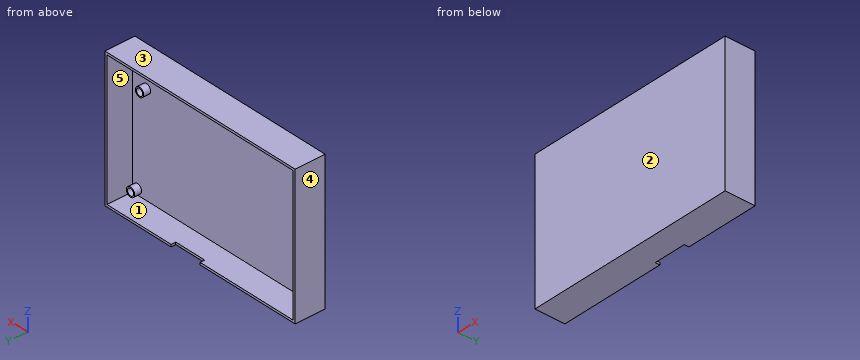
Autodesk Inventor part; units mm, degrees
ref_plane "YZ Plane" through (0, 0, 0) normal (1, 0, 0) x (0, 1, 0)
ref_plane "XZ Plane" through (0, 0, 0) normal (0, 1, 0) x (-1, 0, 0)
ref_plane "XY Plane" through (0, 0, 0) normal (0, 0, 1) x (1, 0, 0)
sketch "Base" plane through (0, 0, 0) normal (0, 1, 0) x (-1, 0, 0)
  line L0 (92, 60.5) -> (-92, 60.5)
  line L1 (-92, 60.5) -> (-92, -60.5)
  line L2 (-92, -60.5) -> (92, -60.5)
  line L3 (92, -60.5) -> (92, 60.5)
  line L4 (92, 60.5) -> (-92, -60.5) construction
  line L5 (-92, 60.5) -> (92, -60.5) construction
  point P0 (0, 0)
  dimension "d0" = 184
  dimension "d1" = 121
extrude "Base - Estrutura" add sketch "Base" against normal blind 26
sketch "Esboço2" plane through (0, 0, 0) normal (0, 1, 0) x (1, 0, 0)
  line L0 (-90, -58.5) -> (90, -58.5)
  line L1 (90, -58.5) -> (90, 58.5)
  line L2 (90, 58.5) -> (-90, 58.5)
  line L3 (-90, 58.5) -> (-90, -58.5)
  line L4 (-90, -58.5) -> (90, 58.5) construction
  line L5 (90, -58.5) -> (-90, 58.5) construction
  point P0 (0, 0)
  dimension "d4" = 180
  dimension "d5" = 117
extrude "Base Interna" cut sketch "Esboço2" against normal blind 22
sketch "Esboço3" plane through (0, -22, 0) normal (0, 1, 0) x (1, 0, 0)
  circle A0 centre (-85, -53.5) radius 4
  line L0 (-92, 60.5) -> (-92, -60.5)
  line L1 (-92, -60.5) -> (92, -60.5)
  circle A1 centre (-85, -53.5) radius 3
  line L2 (-90, -58.5) -> (-90, 58.5)
  line L3 (90, 58.5) -> (90, -58.5)
  circle A2 centre (-85, 53.5) radius 4
  circle A3 centre (-85, 53.5) radius 3
  line L4 (-90, 58.5) -> (90, 58.5)
  line L5 (90, -58.5) -> (-90, -58.5)
  circle A4 centre (85, 53.5) radius 3
  circle A5 centre (85, 53.5) radius 4
  line L6 (92, -60.5) -> (92, 60.5)
  line L7 (92, 60.5) -> (-92, 60.5)
  circle A6 centre (76.27, -28.99) radius 4
  circle A7 centre (76.27, -28.99) radius 3
  point P0 (0, 0)
  dimension "d8" = 8
  dimension "d9" = 7
  dimension "d10" = 7
  dimension "d11" = 6
  dimension "d12" = 7
  dimension "d13" = 7
  dimension "d14" = 8
  dimension "d15" = 31.51
  dimension "d16" = 15.73
  dimension "d17" = 6
  dimension "d29" = 6
  dimension "d30" = 8
  dimension "d31" = 8
  dimension "d32" = 6
extrude "Furos do Pino Guia" add sketch "Esboço3" along normal blind 6 contours A0 | A2 | A5 | A6
sketch "Esboço4" plane through (92, 0, -60.5) normal (0, 0, -1) x (-1, 0, 0)
  line L0 (92, 0) -> (64, 0)
  line L1 (64, 0) -> (64, -4)
  line L2 (64, -4) -> (92, -4)
  line L3 (92, -4) -> (92, 0)
  line L4 (92, 0) -> (64, -4) construction
  line L5 (64, 0) -> (92, -4) construction
  line L6 (184, 0) -> (184, -26)
  line L7 (0, 0) -> (184, 0)
  line L8 (184, -26) -> (0, -26)
  point P0 (92, 0)
  point P1 (78, -2)
  point P2 (64, -2)
  dimension "d20" = 120
  dimension "d21" = 28
  dimension "d22" = 0
  dimension "d24" = 4
extrude "Chaveta para USB-C ESP32" cut sketch "Esboço4" along normal blind 4 and the other way blind 2
properties part number "base_traseira_3DPrint"
Model file for the job. Use its own axes, mm. Face numbers are marked on the shaded views. A direction names the side the tool comes from. Coordinates: 2 decimals unless noted, no trailing zeros. Write each loop counter-clockwise with the first axis right and the second up, starting at its lowest first coordinate (ties: lowest second). Pieces come first, ordered by that corner, then holes. Notation, with made-up numbers: (86.5, 58.5) - (95.5, 58.5) arc R26 cw to (95.5, 78.5) - close; hole circle Ø7 at (-18, 3). An arc over 180 degrees is marked (long way). One line per item, written item: value. Start each with the question number.
1. Slice it at D-D (x = -85). Write the cut outline in (y, z).
2. Probe line 1 (X direction, y = -20.1, z = 28.99); line 2 (Z direction, x = 76.27, y = -19.3); line 3 (X direction, y = -18.05, z = 53.5). List the from-to ranges inside material, lowest first. Write a range as from..to.
3. Flat gauge pins, fed straight in: pin 1 (2 mm diameter, centred on x = 11.5, z = -59, fed in from +Y); pin 2 (6 mm diameter, centred on x = 40.5, z = 9.5, fed in from +Y); pin 3 (6.5 mm diameter, centred on x = -85.5, z = 55, fed in from +Y). Where does each tip first touch, or does it go through?
4. Slice it at B-B (x = 18.5). Write the cut outline in (y, z), plus the area to 3 significant figures.
5. Tool access for the marked faces 1 and 2: list every direction of +Z, -Z, +X, -X, +Y, -Y with a clear straight run to the whole face (end or side of a thin tool).
6. Mould opens along X. For the marked faces 3, 4 and 5 say: released by +X, released by -X, zero draft, split by the parting line, or undercut.
7. Slice it at C-C (z = 53.5). Write the cut outline in (x, y), plus the area to 3 significant figures.
8. Slice it at A-A (y = -10.25). Write the cut outline in (x, z).
Answers below:
1. outline: (-26, -60.5) - (0, -60.5) - (0, -58.5) - (-22, -58.5) - (-22, -57.5) - (-16, -57.5) - (-16, -56.5) - (-22, -56.5) - (-22, -50.5) - (-16, -50.5) - (-16, -49.5) - (-22, -49.5) - (-22, 49.5) - (-16, 49.5) - (-16, 50.5) - (-22, 50.5) - (-22, 56.5) - (-16, 56.5) - (-16, 57.5) - (-22, 57.5) - (-22, 58.5) - (0, 58.5) - (0, 60.5) - (-26, 60.5) - close
2. line 1: x = -92..-90, 72.27..73.27, 79.27..80.27, 90..92
2. line 2: z = -60.5..-58.5, 24.99..25.99, 31.99..32.99, 58.5..60.5
2. line 3: x = -92..-90, -89..-88, -82..-81, 90..92
3. pin 1: stops at y = -4
3. pin 2: stops at y = -22
3. pin 3: stops at y = -16
4. outline: (-26, -60.5) - (-4, -60.5) - (-4, -58.5) - (-22, -58.5) - (-22, 58.5) - (0, 58.5) - (0, 60.5) - (-26, 60.5) - close
4. area: 564 mm^2
5. face 1: +Y
5. face 2: +Z, -Z, +X, -X, -Y
6. face 3: zero draft
6. face 4: released by -X
6. face 5: undercut
7. outline: (-92, -26) - (92, -26) - (92, 0) - (90, 0) - (90, -22) - (-81, -22) - (-81, -16) - (-82, -16) - (-82, -22) - (-88, -22) - (-88, -16) - (-89, -16) - (-89, -22) - (-90, -22) - (-90, 0) - (-92, 0) - close
7. area: 836 mm^2
8. outline: (-92, -60.5) - (92, -60.5) - (92, 60.5) - (-92, 60.5) - close; hole (-90, -58.5) - (90, -58.5) - (90, 58.5) - (-90, 58.5) - close
